Geometry: final body of the model. Coordinates: model frame, mm. A direction names the side the tool comes from. Give positions to 0.01 mm unless a question says otherwise; leave off trailing zeros. Write each loop counter-clockwise with the first axis right and the second up, starting at its lowest first coordinate (ties: lowest second). Pieces come first, ordered by that corner, then holes.
Q1. Line query: line 1 (Y direction, x = -27, z = 13). Output: solid intervals per line, ascending.
Q2. Section C-C (x = -1). Return the cut outline in (y, z), plus the area to 3 significant figures.
Q3. Mould query, pull axis Z, two halves, no side actions, for faces 4 (the flat face through (-8, 17, 0)), 5 (the flat face through (-8, 34, 1)), 6 (the flat face through (-24.236, 1, 18)). Classes: +Z half, -Z half, draft (parallel to the pull), parting line (faces both ways), or undercut.
Q4. Section A-A (y = 18). Return the cut outline in (x, z).
Q5. Section B-B (z = 15.5). Return the cut outline in (x, y), plus the area to 3 significant figures.
Q6. Pin query (flat end, axial travel): pin 1 Ø5 at (x, y) = (0, 18.5) entering from +Z; pin 2 Ø9 at (x, z) = (1.5, 21) entering from +Y; pin 3 Ø4 at (x, y) = (-16.5, 23) entering from +Z. Return the tip coordinate at first contact, or that it passes through.
Q7. Reachability of faces 1 (the flat face through (-8, 18, 2)), 2 (the cylindrical face through (-22.811, 1.014, 5.935)), 3 (the flat face through (15.794, 9.4, 1.7)) from +Z, -Z, +X, -X, +Y, -Y: full face, straight path, thin tool, end or side. Return the list, or none.
Q8. Section D-D (x = -22). Return the cut outline in (y, z).
from build123d import *

# Parameters (mm, degrees)
SKETCH_1_W          = 46
SKETCH_1_H          = 34
EXTRUDE_1_DEPTH     = 2
SKETCH_2_W          = 46
SKETCH_2_H          = 2
EXTRUDE_2_DEPTH     = 30
SKETCH_3_R          = 5.5
CUT_EXTRUDE_1_DEPTH = 2
CUT_EXTRUDE_2_DEPTH = 2


with BuildPart() as part:
    # 草图1 → 凸台-拉伸1 (new body)
    with BuildSketch(Plane.XY):
        with Locations((-7.206275861, 17)):
            Rectangle(SKETCH_1_W, SKETCH_1_H)
    extrude(amount=EXTRUDE_1_DEPTH)

    # 草图2 → 凸台-拉伸2 (add)
    with BuildSketch(Plane.XY.offset(2)):
        with Locations((-7.206275861, 1)):
            Rectangle(SKETCH_2_W, SKETCH_2_H)
    extrude(amount=EXTRUDE_2_DEPTH)

    # 草图3 → 切除-拉伸1 (cut)
    with BuildSketch(Plane.XY.offset(2)):
        with Locations((-17.206275861, 18)):
            Circle(SKETCH_3_R)
        with Locations((2.793724139, 18)):
            Circle(SKETCH_3_R)
    extrude(amount=-CUT_EXTRUDE_1_DEPTH, mode=Mode.SUBTRACT)

    # 草图4 → 切除-拉伸2 (cut)
    with BuildSketch(Plane(origin=(0, 2, 0), x_dir=(1, 0, 0), z_dir=(0, 1, 0))):
        with BuildLine():
            Line((-24.235699599, -7.328343443), (-24.235699599, -28.539953108))
            ThreePointArc((-24.235699599, -28.539953108), (-22.841637624, -29.934015083), (-21.447575649, -28.539953108))
            Line((-21.447575649, -28.539953108), (-21.447575649, -7.328343443))
            ThreePointArc((-21.447575649, -7.328343443), (-22.841637624, -5.934281468), (-24.235699599, -7.328343443))
        make_face()
        with BuildLine():
            Line((7.035023927, -7.328343443), (7.035023927, -28.539953108))
            ThreePointArc((7.035023927, -28.539953108), (8.429085903, -29.934015083), (9.823147878, -28.539953108))
            Line((9.823147878, -28.539953108), (9.823147878, -7.328343443))
            ThreePointArc((9.823147878, -7.328343443), (8.429085903, -5.934281468), (7.035023927, -7.328343443))
        make_face()
    extrude(amount=-CUT_EXTRUDE_2_DEPTH, mode=Mode.SUBTRACT)


solid = part.part
Computed:
1. line 1: y = 0 to 2
2. outline: (0, 0) - (14.02, 0) - (14.02, 2) - (2, 2) - (2, 32) - (0, 32) - close; (21.98, 0) - (34, 0) - (34, 2) - (21.98, 2) - close
2. area: 112 mm2
3. face 4: -Z half
3. face 5: draft
3. face 6: undercut
4. outline: (-30.21, 0) - (-22.71, 0) - (-22.71, 2) - (-30.21, 2) - close; (-11.71, 0) - (-2.71, 0) - (-2.71, 2) - (-11.71, 2) - close; (8.29, 0) - (15.79, 0) - (15.79, 2) - (8.29, 2) - close
5. outline: (-30.21, 0) - (-24.24, 0) - (-24.24, 2) - (-30.21, 2) - close; (-21.45, 0) - (7.04, 0) - (7.04, 2) - (-21.45, 2) - close; (9.82, 0) - (15.79, 0) - (15.79, 2) - (9.82, 2) - close
5. area: 80.8 mm2
6. pin 1: passes through
6. pin 2: stops at y = 2
6. pin 3: stops at z = 2
7. face 1: +Z, +X, -X, +Y
7. face 2: +Y, -Y
7. face 3: +Z, -Z, +X, +Y, -Y
8. outline: (0, 0) - (15.3, 0) - (15.3, 2) - (2, 2) - (2, 6.22) - (0, 6.22) - close; (0, 29.65) - (2, 29.65) - (2, 32) - (0, 32) - close; (20.7, 0) - (34, 0) - (34, 2) - (20.7, 2) - close
